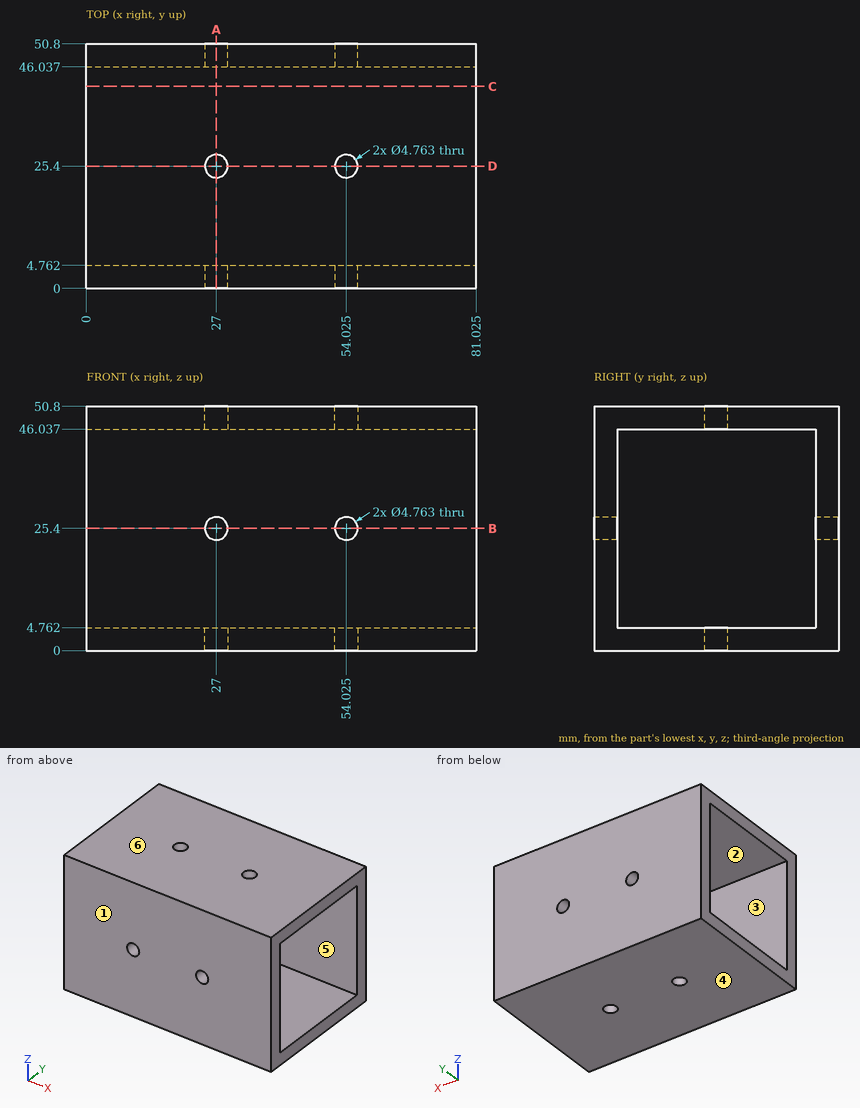
Job drawing, mm, ordinate dimensions from the low corner. One solid piece. A direction names the side the tool comes from. Coordinates: 2 decimals unless noted, no trailing zeros. Write each loop counter-clockwise with the first axis right and the second up, starting at its lowest first coordinate (ties: lowest second). Pieces come first, ordered by that corner, then holes. Notation, with made-up numbers: M -39,42 L -3,42 A13 ccw -3,63 Z; hole C -3.5,52.25 d11. An arc over 180 degrees is marked long. Answer as a JSON object with one key per item and string values. Group by question number.
1) Tool access for the marked faces 5 and 6: list every direction of +Z, -Z, +X, -X, +Y, -Y with a clear straight run to the whole face (end or side of a thin tool).
2) Mould opens along Z. For the marked faces 1, 2, 3 and 4 say: +Z half, -Z half, draft (parallel to the pull), parting line (faces both ways), or undercut.
3) Pin check, flat tip, straight feed: pin 1 Ø1 at (x, z) = (46, 18) entering from -Y. Stop position of the tip, or through.
4) Saw through at A-A (x = 27). Write the cut outline in (y, z).
5) Saw through at C-C (y = 42). Write the cut outline in (x, z) (1 decimal).
6) Saw through at B-B (z = 25.4). Write the cut outline in (x, y) (1 decimal), plus the area to 3 significant figures.
7) Wall check: line 1 (Y direction, x = 35.5, z = 12.5); line 2 (Y direction, x = 27, z = 3). Give the ranges that are in metal, low to high. Write a range as from..to.
Values follow:
{
 "1": {"face 5": "+X, -X", "face 6": "+Z, +X, -X, +Y, -Y"},
 "2": {"face 1": "draft", "face 2": "undercut", "face 3": "undercut", "face 4": "-Z half"},
 "3": {"pin 1": "stops at y = 0"},
 "4": {"outline": "M 0,0 L 23.02,0 L 23.02,4.76 L 4.76,4.76 L 4.76,23.02 L 0,23.02 Z; M 0,27.78 L 4.76,27.78 L 4.76,46.04 L 23.02,46.04 L 23.02,50.8 L 0,50.8 Z; M 27.78,0 L 50.8,0 L 50.8,23.02 L 46.04,23.02 L 46.04,4.76 L 27.78,4.76 Z; M 27.78,46.04 L 46.04,46.04 L 46.04,27.78 L 50.8,27.78 L 50.8,50.8 L 27.78,50.8 Z"},
 "5": {"outline": "M 0,0 L 81,0 L 81,4.8 L 0,4.8 Z; M 0,46 L 81,46 L 81,50.8 L 0,50.8 Z"},
 "6": {"outline": "M 0,0 L 24.6,0 L 24.6,4.8 L 0,4.8 Z; M 0,46 L 24.6,46 L 24.6,50.8 L 0,50.8 Z; M 29.4,0 L 51.6,0 L 51.6,4.8 L 29.4,4.8 Z; M 29.4,46 L 51.6,46 L 51.6,50.8 L 29.4,50.8 Z; M 56.4,0 L 81,0 L 81,4.8 L 56.4,4.8 Z; M 56.4,46 L 81,46 L 81,50.8 L 56.4,50.8 Z", "area": "681 mm2"},
 "7": {"line 1": "y = 0..4.76, 46.04..50.8", "line 2": "y = 0..23.02, 27.78..50.8"}
}
